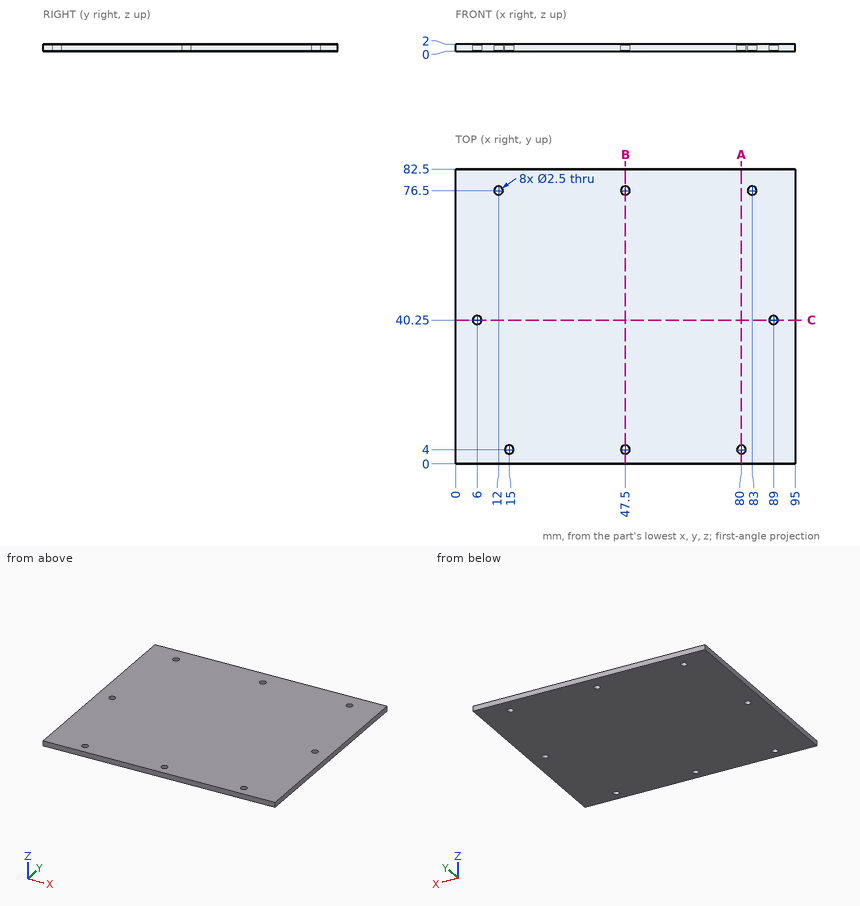
Geometry: see drawing. Coordinates: mm, zero at the bounding-box minimum. Give positions to 0.01 mm unless a question says otherwise; leave off trailing zeros. Write each loop counter-clockwise with the first axis right and the second up, starting at its lowest first coordinate (ties: lowest second). Pieces come first, ordered by that corner, then holes. Notation, with made-up numbers: M 5.5,-22 L 64.5,-22 A29 cw 64.5,16 Z; hole C 81.25,48 d11. An arc over 180 degrees is marked long. Answer as a JSON object with one key per item and string values.
Q1. Cut plane B-B, the plane x = 47.5. Return the cut outline in (y, z).
Geometry check:
{"outline": "M 0,0 L 2.75,0 L 2.75,2 L 0,2 Z; M 5.25,0 L 75.25,0 L 75.25,2 L 5.25,2 Z; M 77.75,0 L 82.5,0 L 82.5,2 L 77.75,2 Z"}
Q2. Cut plane A-A, the plane x = 80. Return the cut outline in (y, z).
Geometry check:
{"outline": "M 0,0 L 2.75,0 L 2.75,2 L 0,2 Z; M 5.25,0 L 82.5,0 L 82.5,2 L 5.25,2 Z"}
Q3. Ray query, line 1 along Y through (x, z) = (47.5, 1.65); line 2 along X through (y, z) = (76.5, 0.9); line 3 along Y through (x, z) = (6, 0.95). Return the intervals inside material, ascending.
Geometry check:
{"line 1": "y = 0 to 2.75, 5.25 to 75.25, 77.75 to 82.5", "line 2": "x = 0 to 10.75, 13.25 to 46.25, 48.75 to 81.75, 84.25 to 95", "line 3": "y = 0 to 39, 41.5 to 82.5"}
Q4. Cut plane C-C, the plane y = 40.25. Return the cut outline in (x, z).
Geometry check:
{"outline": "M 0,0 L 4.75,0 L 4.75,2 L 0,2 Z; M 7.25,0 L 87.75,0 L 87.75,2 L 7.25,2 Z; M 90.25,0 L 95,0 L 95,2 L 90.25,2 Z"}
